```python
from build123d import *

# Parameters (mm, degrees)
SKETCH_W        = 150
SKETCH_H        = 30
PAD_DEPTH       = 5
SKETCH001_W     = 150
SKETCH001_H     = 5
PAD001_DEPTH    = 40
SKETCH002_R     = 14.5
SKETCH002_R_2   = 7.75
POCKET_DEPTH    = 30.001
FILLET_R        = 10
SKETCH003_W     = 10
SKETCH003_H     = 6
PAD002_DEPTH    = 3
SKETCH004_R     = 3
POCKET001_DEPTH = 8.001
SKETCH005_W     = 5
SKETCH005_H     = 20
PAD003_DEPTH    = 20
CHAMFER_SIZE    = 18
FILLET001_R     = 2


with BuildPart() as part:
    # Sketch → Pad (new body)
    with BuildSketch(Plane.XY):
        with Locations((75, 15)):
            Rectangle(SKETCH_W, SKETCH_H)
    extrude(amount=PAD_DEPTH)

    # Sketch001 (on Face6 of Pad) → Pad001 (join)
    with BuildSketch(Plane.XY.offset(5)):
        with Locations((75, 2.5)):
            Rectangle(SKETCH001_W, SKETCH001_H)
    extrude(amount=PAD001_DEPTH)

    # Sketch002 (on Face5 of Pad001) → Pocket (cut, through all)
    with BuildSketch(Plane.XZ):
        with Locations((20, 25)):
            Circle(SKETCH002_R)
        with Locations((75, 25)):
            Circle(SKETCH002_R)
        with Locations((130, 25)):
            Circle(SKETCH002_R_2)
    extrude(amount=-POCKET_DEPTH, mode=Mode.SUBTRACT)

    # Fillet
    fillet_edges = [part.edges().sort_by_distance(p)[0] for p in [
        (150, 2.5, 45),
        (0, 2.5, 45),
    ]]
    fillet(fillet_edges, radius=FILLET_R)

    # Sketch003 → Pad002 (join)
    with BuildSketch(Plane(origin=(0, 0, 0), x_dir=(1, 0, 0), z_dir=(0, 0, -1))):
        with Locations((5, -15)):
            Rectangle(SKETCH003_W, SKETCH003_H)
        with Locations((145, -15)):
            Rectangle(SKETCH003_W, SKETCH003_H)
    extrude(amount=PAD002_DEPTH)

    # Sketch004 (on Face15 of Pad002) → Pocket001 (cut, through all)
    with BuildSketch(Plane.XY.offset(5)):
        with Locations((75, 15)):
            Circle(SKETCH004_R)
    extrude(amount=-POCKET001_DEPTH, mode=Mode.SUBTRACT)

    # Sketch005 (on Face15 of Pocket001) → Pad003 (join)
    with BuildSketch(Plane.XY.offset(5)):
        with Locations((47.5, 15)):
            Rectangle(SKETCH005_W, SKETCH005_H)
        with Locations((105.875, 15)):
            Rectangle(SKETCH005_W, SKETCH005_H)
    extrude(amount=PAD003_DEPTH)

    # Chamfer
    chamfer_edges = [part.edges().sort_by_distance(p)[0] for p in [
        (105.875, 25, 25),
        (47.5, 25, 25),
    ]]
    chamfer(chamfer_edges, length=CHAMFER_SIZE)

    # Fillet001
    fillet001_edges = [part.edges().sort_by_distance(p)[0] for p in [
        (129.1875, 5, 5),
        (76.6875, 5, 5),
        (22.5, 5, 5),
    ]]
    fillet(fillet001_edges, radius=FILLET001_R)


solid = part.part
```
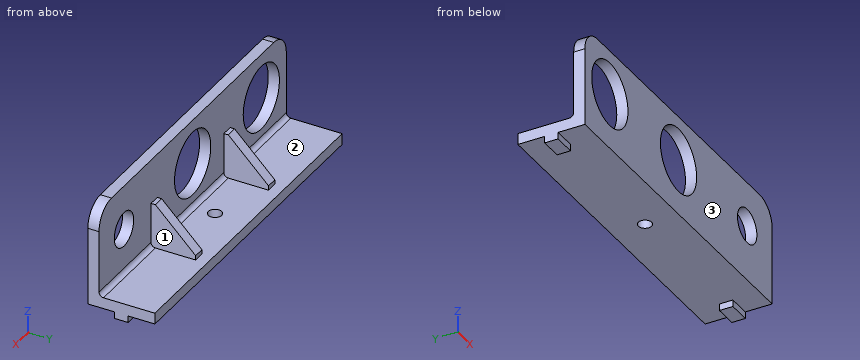
Input: part model. Units: mm. Frame: model coordinates. Face numbers are marked on the shaded views. Coordinates: 2 decimals unless noted, no trailing zeros. Write each loop counter-clockwise with the first axis right and the second up, starting at its lowest first coordinate (ties: lowest second). Pieces come first, ordered by that corner, then holes. Notation, with made-up numbers: M -5.5,63.25 L 6.5,63.25 A24 cw 6.5,99.25 Z; hole C 38.25,61.25 d2. An arc over 180 degrees is marked long. Use one line per item in the form item = value.
Q1. Section C-C (x = 130). Return loops of the section in (y, z).
Answer below:
outline = M 0,0 L 30,0 L 30,5 L 7,5 A2 cw 5,7 L 5,17.25 L 0,17.25 Z; M 0,32.75 L 5,32.75 L 5,45 L 0,45 Z
Q2. First-contact query: pin 1 (12 mm diameter, centred on x = 83.5, y = 12.5, fed in from -Z); pin 2 (12.5 mm diameter, centred on x = 130, z = 25, fed in from +Y); pin 3 (9.5 mm diameter, centred on x = 75, y = 15, fed in from +Z); pin 4 (0.9 mm diameter, centred on x = 146, z = -2, fed in from -Y). Flat tips, straight axial feed; report the tip coordinate or a pass-through.
Answer below:
pin_1 = 0
pin_2 = through
pin_3 = 5
pin_4 = 12
Q3. Section B-B (y = 15). Return loops of the section in (x, z) (3 decimals), plus the area to 3 significant figures.
Answer below:
outline = M 0,-3 L 10,-3 L 10,0 L 72,0 L 72,5 L 50,5 L 50,17 L 45,17 L 45,5 L 0,5 Z; M 78,0 L 140,0 L 140,-3 L 150,-3 L 150,5 L 108.375,5 L 108.375,17 L 103.375,17 L 103.375,5 L 78,5 Z
area = 900 mm²
Q4. Draft query along X for the marked faces 1, 2 and 3. Return one class per face: released by +X, released by -X, zero draft, split by the parting line, or undercut.
Answer below:
face_1 = released by +X
face_2 = undercut
face_3 = zero draft
Q5. Section D-D (z = 13). Return loops of the section in (x, y) (3 decimals), plus the area to 3 significant figures.
Answer below:
outline = M 0,0 L 11.861,0 L 11.861,5 L 0,5 Z; M 28.139,0 L 66.861,0 L 66.861,5 L 50,5 L 50,19 L 45,19 L 45,5 L 28.139,5 Z; M 83.139,0 L 150,0 L 150,5 L 108.375,5 L 108.375,19 L 103.375,19 L 103.375,5 L 83.139,5 Z
area = 727 mm²
Q6. Section A-A (x = 75). Return loops of the section in (y, z), plus the area to 3 significant figures.
Answer below:
outline = M 0,0 L 12,0 L 12,5 L 7,5 A2 cw 5,7 L 5,10.5 L 0,10.5 Z; M 0,39.5 L 5,39.5 L 5,45 L 0,45 Z; M 18,0 L 30,0 L 30,5 L 18,5 Z
area = 176 mm²
Q7. Material intervals for probe 1 along X at (y, z) = (2.5, 23); probe 2 along Y at (x, z) = (75, 2); probe 3 along Z at (x, y) = (75, 2.35), sorted ascending. Write a range as from..to.
Answer below:
probe_1 = 0..5.64, 34.36..60.64, 89.36..122.51, 137.49..150
probe_2 = 0..12, 18..30
probe_3 = 0..10.5, 39.5..45
